from build123d import *

# Parameters (mm, degrees)
F0_W      = 25
F0_H      = 80
F1_DEPTH  = 10
F2_W      = 25
F2_H      = 10
F3_DEPTH  = 45
F4_R      = 2
F4_R_2    = 1.5
F5_DEPTH  = 10.001
F6_R      = 1.5
F7_DEPTH  = 6
F8_R      = 1.5
F8_R_2    = 2
F9_DEPTH  = 10.001
F10_R     = 2
F11_DEPTH = 10


with BuildPart() as f1:
    # F0 (on Front) → F1 (new body)
    with BuildSketch(Plane.XZ):
        Rectangle(F0_W, F0_H)
    extrude(amount=F1_DEPTH)

    # F2 (on face) → F3 (join)
    with BuildSketch(Plane.XZ.offset(10)):
        with Locations((0, -35)):
            Rectangle(F2_W, F2_H)
    extrude(amount=F3_DEPTH)

    # F4 (on face) → F5 (cut, through all)
    with BuildSketch(Plane.XZ.offset(10)):
        with Locations((-7.5, 26)):
            Circle(F4_R)
        with Locations((0, -17.5)):
            Circle(F4_R_2)
        with Locations((0, 2.5)):
            Circle(F4_R_2)
        with Locations((0, 22.5)):
            Circle(F4_R_2)
        with Locations((6, 22.5)):
            Circle(F4_R_2)
        with Locations((6, -17.5)):
            Circle(F4_R_2)
    extrude(amount=-F5_DEPTH, mode=Mode.SUBTRACT)

    # F6 (on face) → F7 (cut)
    with BuildSketch(Plane.YZ.offset(12.5)):
        with Locations((-5, 36)):
            Circle(F6_R)
    extrude(amount=-F7_DEPTH, mode=Mode.SUBTRACT)

    # F8 (on face) → F9 (cut, through all)
    with BuildSketch(Plane.XY.offset(-30)):
        with Locations((0, -36)):
            Circle(F8_R)
        with Locations((0, -24)):
            Circle(F8_R_2)
        with Locations((-7, -36)):
            Circle(F8_R)
        with Locations((7, -36)):
            Circle(F8_R)
        with Locations((0, -50)):
            Circle(F8_R)
        with Locations((-7, -50)):
            Circle(F8_R)
        with Locations((7, -50)):
            Circle(F8_R)
    extrude(amount=-F9_DEPTH, mode=Mode.SUBTRACT)

    # F10 (on face) → F11 (cut)
    with BuildSketch(Plane(origin=(-12.5, 0, 0), x_dir=(0, -1, 0), z_dir=(-1, 0, 0))):
        with Locations((5, -35)):
            Circle(F10_R)
        with Locations((15, -35)):
            Circle(F10_R)
    extrude(amount=-F11_DEPTH, mode=Mode.SUBTRACT)


solid = f1.part
CAD build for the part. Positions are in the model's coordinates, mm. A direction names the side the tool comes from. Round coordinates to 2 decimals unless told otherwise and drop trailing zeros. Write each loop counter-clockwise with the first axis right and the second up, starting at its lowest first coordinate (ties: lowest second). Pieces come first, ordered by that corner, then holes.
(1) Slice it at B-B, the plane y = -24. Write the cut outline in (x, z).
(2) Slice it at A-A, the plane z = 26. Write the cut outline in (x, y), and give its area (3 significant figures).
(3) Drop flat-ended pins along their axis: P1, Ø2.5, axis at x = -7, y = -36, coming from the -Z side; P2, Ø3, axis at y = -5, z = -35, coming from the -X side; P3, Ø1.5, axis at y = -4.5, z = 36.5, coming from the +X side; P4, Ø3, axis at x = -8.5, y = -18, coming from the +Z side. Give the stop position or say it passes through.
(4) Probe line 1 along Z through (x, y) = (6, -4.25); line 2 along Y through (x, z) = (7, -33); line 3 along Z through (x, y) = (-9.5, -15). List the from-to ranges inside material, lowest first.
(5) Slice it at D-D, the plane z = -17.5. Write the cut outline in (x, y), and give its area (3 significant figures).
(6) 3-axis set-ups, long thin cutter, end or side, ignore diameter. For faces 1 (the face through (-8, -5, -37)), 2 (the face through (0, -5, -16)), 3 (the face through (9.542, -5.325, 34.536)): which of +Z, -Z, +X, -X, +Y, -Y reach the whole face in a straight line?
(7) Slice it at C-C, the plane x = 9.5. Write the cut outline in (y, z).
(8) Mould opens along Z. For faces 4 (the face through (0, -32, -30)), 5 (the face through (-2.5, -5, -35)), 6 (the face through (-12.5, -9, -12)) say: pulls with the +Z half, pulls with the -Z half, needs draft (parallel to the pull), parting line crosses it, or undercut.
From the geometry:
1. outline: (-12.5, -40) - (-2, -40) - (-2, -30) - (-12.5, -30) - close; (2, -40) - (12.5, -40) - (12.5, -30) - (2, -30) - close
2. outline: (-12.5, -10) - (-9.5, -10) - (-9.5, 0) - (-12.5, 0) - close; (-5.5, -10) - (12.5, -10) - (12.5, 0) - (-5.5, 0) - close
2. area: 210 mm2
3. P1: passes through
3. P2: stops at x = -2.5
3. P3: stops at x = 6.5
3. P4: stops at z = -30
4. line 1: z = -40 to -19, -16 to 21, 24 to 40
4. line 2: y = -55 to -51.5, -48.5 to -37.5, -34.5 to 0
4. line 3: z = -40 to -37, -33 to -30
5. outline: (-12.5, -10) - (-1.5, -10) - (-1.5, 0) - (-12.5, 0) - close; (1.5, -10) - (4.5, -10) - (4.5, 0) - (1.5, 0) - close; (7.5, -10) - (12.5, -10) - (12.5, 0) - (7.5, 0) - close
5. area: 190 mm2
6. face 1: -X
6. face 2: +Y, -Y
6. face 3: +X
7. outline: (-55, -40) - (0, -40) - (0, 40) - (-10, 40) - (-10, -30) - (-55, -30) - close; hole circle Ø3 at (-5, 36)
8. face 4: pulls with the +Z half
8. face 5: undercut
8. face 6: needs draft
